```python
from build123d import *

# Parameters (mm, degrees)
F0_W         = 16
F0_H         = 36
F1_DEPTH     = 4
F2_DEPTH     = 3
F3_W         = 4.8
F3_H         = 1.6
F4_DEPTH     = 20.1
F5_T1_DEPTH  = 5.5
F5_T3_DEPTH  = 6
F5_T6_ANGLE  = 90
F5_T8_ANGLE  = 90
F5_T10_ANGLE = 90
F5_T12_ANGLE = 90
F6_T1_DEPTH  = 4.8
F7_R         = 1


# Not quite as in the source:
# - a fillet or chamfer that OpenCascade refuses, or shapes differently, is made with other operations: its cross-section is extruded or revolved along the edge and cut away or added


with BuildPart() as f1:
    # F0 (on Top) → F1 (new body)
    with BuildSketch(Plane.XY):
        with BuildLine():
            ThreePointArc((10, 17), (9.1213203436, 19.1213203436), (7, 20))
            Line((7, 20), (-7, 20))
            ThreePointArc((-7, 20), (-9.1213203436, 19.1213203436), (-10, 17))
            Line((-10, 17), (-10, -17))
            ThreePointArc((-10, -17), (-9.1213203436, -19.1213203436), (-7, -20))
            Line((-7, -20), (7, -20))
            ThreePointArc((7, -20), (9.1213203436, -19.1213203436), (10, -17))
            Line((10, -17), (10, -9))
            ThreePointArc((10, -9), (10.8786796564, -6.8786796564), (13, -6))
            Line((13, -6), (17, -6))
            ThreePointArc((17, -6), (19.1213203436, -5.1213203436), (20, -3))
            Line((20, -3), (20, 3))
            ThreePointArc((20, 3), (19.1213203436, 5.1213203436), (17, 6))
            Line((17, 6), (13, 6))
            ThreePointArc((13, 6), (10.8786796564, 6.8786796564), (10, 9))
            Line((10, 9), (10, 17))
        make_face()
        Rectangle(F0_W, F0_H, mode=Mode.SUBTRACT)
        with BuildLine():
            ThreePointArc((10.1, 2.75), (10.3928932188, 3.4571067812), (11.1, 3.75))
            Line((11.1, 3.75), (17.1, 3.75))
            ThreePointArc((17.1, 3.75), (17.8071067812, 3.4571067812), (18.1, 2.75))
            Line((18.1, 2.75), (18.1, -2.75))
            ThreePointArc((18.1, -2.75), (17.8071067812, -3.4571067812), (17.1, -3.75))
            Line((17.1, -3.75), (11.1, -3.75))
            ThreePointArc((11.1, -3.75), (10.3928932188, -3.4571067812), (10.1, -2.75))
            Line((10.1, -2.75), (10.1, 2.75))
        make_face(mode=Mode.SUBTRACT)
    extrude(amount=F1_DEPTH)

    # F0 (on Top) → F2 (join)
    with BuildSketch(Plane.XY):
        Rectangle(F0_W, F0_H)
    extrude(amount=F2_DEPTH)

    # F3 (on face) → F4 (cut, through all)
    with BuildSketch(Plane(origin=(-10, 0, 0), x_dir=(0, -1, 0), z_dir=(-1, 0, 0))):
        with Locations((0, 1.6)):
            Rectangle(F3_W, F3_H)
    extrude(amount=-F4_DEPTH, mode=Mode.SUBTRACT)

    # F5: chamfer of 1 on 1 edges, made by hand

    # F5_s2 → F5_t1 (cut)
    with BuildSketch(Plane.XZ.offset(-2.75)):
        Polygon((19.1, 0), (18.1, 1), (18.1, 0), align=None)
        Polygon((9.1, 0), (10.1, 1), (10.1, 0), align=None)
    extrude(amount=F5_T1_DEPTH, mode=Mode.SUBTRACT)

    # F5_s4 → F5_t3 (cut)
    with BuildSketch(Plane.YZ.offset(11.1)):
        Polygon((-4.75, 0), (-3.75, 1), (-3.75, 0), align=None)
        Polygon((4.75, 0), (3.75, 1), (3.75, 0), align=None)
    extrude(amount=F5_T3_DEPTH, mode=Mode.SUBTRACT)

    # F5_s5 → F5_t6 (revolve, cut)
    with BuildSketch(Plane.YZ.offset(17.1)):
        Polygon((4.75, 0), (3.75, 1), (3.75, 0), align=None)
    revolve(axis=Axis((17.1, 2.75, 0), (0, 0, -1)), revolution_arc=F5_T6_ANGLE, mode=Mode.SUBTRACT)

    # F5_s7 → F5_t8 (revolve, cut)
    with BuildSketch(Plane.XZ.offset(2.75)):
        Polygon((19.1, 0), (18.1, 1), (18.1, 0), align=None)
    revolve(axis=Axis((17.1, -2.75, 0), (0, 0, -1)), revolution_arc=F5_T8_ANGLE, mode=Mode.SUBTRACT)

    # F5_s9 → F5_t10 (revolve, cut)
    with BuildSketch(Plane.YZ.offset(11.1)):
        Polygon((-4.75, 0), (-3.75, 1), (-3.75, 0), align=None)
    revolve(axis=Axis((11.1, -2.75, 0), (0, 0, -1)), revolution_arc=F5_T10_ANGLE, mode=Mode.SUBTRACT)

    # F5_s11 → F5_t12 (revolve, cut)
    with BuildSketch(Plane.XZ.offset(-2.75)):
        Polygon((9.1, 0), (10.1, 1), (10.1, 0), align=None)
    revolve(axis=Axis((11.1, 2.75, 0), (0, 0, -1)), revolution_arc=F5_T12_ANGLE, mode=Mode.SUBTRACT)

    # F6: fillet of radius 1 on 1 edges, made by hand

    # F6_s2 → F6_t1 (cut)
    with BuildSketch(Plane.XZ.offset(-2.4)):
        with BuildLine():
            ThreePointArc((8.1928932188, -0.9071067812), (8.4096659701, 0.1826834324), (7.4857864376, 0.8))
            Line((7.4857864376, 0.8), (9.9, 0.8))
            Line((9.9, 0.8), (8.1928932188, -0.9071067812))
        make_face()
    extrude(amount=F6_T1_DEPTH, mode=Mode.SUBTRACT)

    # F7
    f7_edges = [f1.edges().sort_by_distance(p)[0] for p in [
        (-10, 0, 4),
    ]]
    fillet(f7_edges, radius=F7_R)


solid = f1.part
```
Work out the finished part from the listing and answer in its coordinate system (mm). A direction names the side the tool comes from. Coordinates: 2 decimals unless noted, no trailing zeros. Loops run counter-clockwise (first coordinate to the right, second up) from the corner with the lowest first, then second, coordinate; pieces in that order, holes last. Notation, with made-up numbers: (-12, 60) -> (47, 60) arc R16 ccw to (47, 72) -> close; hole circle Ø2 at (-30.5, 7.25). An arc over 180 degrees is marked (long way). Answer as CSV lines item,"result".
Q1. A tool of negligible diameter and unlimited length cuts with its end or side. For faces 1 (the face through (10.401, -3.465, 2.479)), 2 (the face through (9.1, -19.14, 1.48)), 3 (the face through (-9.699, -0.238, 3.715)), 4 (the face through (-8, -0.3, 3.5)), 5 (the face through (8.126, 0.034, 0.568)), from which of +Z, -Z, +X, -X, +Y, -Y can it reach the whole face along a straight path? Write none if from no direction.
Findings:
face 1,"+Z, -Z"
face 2,"+Z, -Z, +X, -Y"
face 3,"+Z, -X, +Y, -Y"
face 4,"+Z"
face 5,"none"
Q2. Each of these flat-tipped pins is pushed along its axis until it touches: pin 1 (0.8 mm diameter, centred on x = 2.5, z = 3.5, fed in from -Y) (3 decimals); pin 2 (5.5 mm diameter, centred on x = -1.5, y = 0, fed in from +Z); pin 3 (0.9 mm diameter, centred on x = 15.5, z = 2, fed in from -Y). Where does it stop, or does it pass through?
Findings:
pin 1,"stops at y = -19.995"
pin 2,"stops at z = 3"
pin 3,"stops at y = -6"
Q3. The part is cut by section B-B on y = 0. Write down the section's boundary in (x, z), and give its area (3 significant figures).
Findings:
outline,"(-10, 0) -> (8.47, 0) arc R1 ccw to (7.49, 0.8) -> (-10, 0.8) -> close; (-10, 2.4) -> (10.1, 2.4) -> (10.1, 4) -> (8, 4) -> (8, 3) -> (-8, 3) -> (-8, 4) -> (-9, 4) arc R1 ccw to (-10, 3) -> close; (18.1, 1) -> (19.1, 0) -> (20, 0) -> (20, 3) arc R1 ccw to (19, 4) -> (18.1, 4) -> close"
area,"37.4 mm²"
Q4. The part is cut by section C-C on x = 13.5. Write down the section's boundary in (y, z).
Findings:
outline,"(-6, 0) -> (-4.75, 0) -> (-3.75, 1) -> (-3.75, 4) -> (-5, 4) arc R1 ccw to (-6, 3) -> close; (3.75, 1) -> (4.75, 0) -> (6, 0) -> (6, 3) arc R1 ccw to (5, 4) -> (3.75, 4) -> close"
Q5. The part is cut by section D-D on z = 1.6. Write down the section's boundary in (x, y).
Findings:
outline,"(-10, -17) arc R3 ccw to (-7, -20) -> (7, -20) arc R3 ccw to (10, -17) -> (10, -9) arc R3 cw to (13, -6) -> (17, -6) arc R3 ccw to (20, -3) -> (20, 3) arc R3 ccw to (17, 6) -> (13, 6) arc R3 cw to (10, 9) -> (10, 17) arc R3 ccw to (7, 20) -> (-7, 20) arc R3 ccw to (-10, 17) -> (-10, 2.4) -> (10.1, 2.4) -> (10.1, 2.75) arc R1 cw to (11.1, 3.75) -> (17.1, 3.75) arc R1 cw to (18.1, 2.75) -> (18.1, -2.75) arc R1 cw to (17.1, -3.75) -> (11.1, -3.75) arc R1 cw to (10.1, -2.75) -> (10.1, -2.4) -> (-10, -2.4) -> close"
Q6. The part is cut by section A-A on x = -2.5. Write down the section's boundary in (y, z).
Findings:
outline,"(-20, 0) -> (20, 0) -> (20, 3) arc R1 ccw to (19, 4) -> (18, 4) -> (18, 3) -> (-18, 3) -> (-18, 4) -> (-19, 4) arc R1 ccw to (-20, 3) -> close; hole (-2.4, 0.8) -> (2.4, 0.8) -> (2.4, 2.4) -> (-2.4, 2.4) -> close"
Q7. Find the intervals of material crossed by probe 1 along Y at (x, z) = (14.5, 1.5); probe 2 along Z at (x, y) = (4.5, -2); probe 3 along Y at (x, z) = (-6.5, 1.3), in increasing order.
Findings:
probe 1,"y = -6 to -3.75, 3.75 to 6"
probe 2,"z = 0 to 0.8, 2.4 to 3"
probe 3,"y = -20 to -2.4, 2.4 to 20"
Q8. For a pull along Z with two mould halves and no side action, classify faces 6 (the face through (0, 2.4, 1)), 7 (the face through (10.112, 3.716, 0.618)), 8 (the face through (-1, 0, 0.8)), 9 (the face through (8, -0.3, 3.5)) as +Z half, -Z half, draft (parallel to the pull), parting line (faces both ways), or undercut.
Findings:
face 6,"undercut"
face 7,"-Z half"
face 8,"undercut"
face 9,"draft"
